```python
from build123d import *

# Parameters (mm, degrees)
F0_W     = 254
F0_H     = 25.0825
F1_DEPTH = 3.175
F2_DEPTH = 22.225
F3_DEPTH = 25.4


# Not quite as in the source:
# - a feature names something its author has since deleted; it is built from what else it names


with BuildPart() as f1:
    # F0 (on Top) → F1 (new body)
    with BuildSketch(Plane.XY):
        with Locations((-10.5066807906, 37.553641122)):
            Rectangle(F0_W, F0_H)
    extrude(amount=F1_DEPTH)



with BuildPart() as f1b:
    # F0 (on Top) → F1, piece 2 (new body)
    with BuildSketch(Plane.XY):
        with Locations((-10.5066807906, 7.391141122)):
            Rectangle(F0_W, F0_H)
    extrude(amount=F1_DEPTH)


with BuildPart() as f1c:
    # F0 (on Top) → F1, piece 3 (new body)
    with BuildSketch(Plane.XY):
        Polygon((-137.5066807906, -61.030108878), (-137.5066807906, -66.110108878), (-112.1066807906, -66.110108878), (-112.1066807906, -61.030108878), (-112.1066807906, -10.230108878), (-137.5066807906, -10.230108878), align=None)
    extrude(amount=F1_DEPTH)


with BuildPart() as f1d:
    # F0 (on Top) → F1, piece 4 (new body)
    with BuildSketch(Plane.XY):
        Polygon((-107.0266807906, -61.030108878), (-107.0266807906, -66.110108878), (-81.6266807906, -66.110108878), (-81.6266807906, -61.030108878), (-81.6266807906, -10.230108878), (-107.0266807906, -10.230108878), align=None)
    extrude(amount=F1_DEPTH)


with BuildPart() as f1e:
    # F0 (on Top) → F1, piece 5 (new body)
    with BuildSketch(Plane.XY):
        Polygon((-76.5466807906, -61.030108878), (-76.5466807906, -66.110108878), (-51.1466807906, -66.110108878), (-51.1466807906, -61.030108878), (-51.1466807906, -10.230108878), (-76.5466807906, -10.230108878), align=None)
    extrude(amount=F1_DEPTH)


with BuildPart() as f1f:
    # F0 (on Top) → F1, piece 6 (new body)
    with BuildSketch(Plane.XY):
        Polygon((-46.0666807906, -61.030108878), (-46.0666807906, -66.110108878), (-20.6666807906, -66.110108878), (-20.6666807906, -61.030108878), (-20.6666807906, -10.230108878), (-46.0666807906, -10.230108878), align=None)
    extrude(amount=F1_DEPTH)


with BuildPart() as f1g:
    # F0 (on Top) → F1, piece 7 (new body)
    with BuildSketch(Plane.XY):
        Polygon((-15.5866807906, -66.110108878), (9.8133192094, -66.110108878), (9.8133192094, -61.030108878), (9.8133192094, -10.230108878), (-15.5866807906, -10.230108878), (-15.5866807906, -61.030108878), align=None)
    extrude(amount=F1_DEPTH)


with BuildPart() as f1h:
    # F0 (on Top) → F1, piece 8 (new body)
    with BuildSketch(Plane.XY):
        Polygon((14.8933192094, -66.110108878), (40.2933192094, -66.110108878), (40.2933192094, -61.030108878), (40.2933192094, -10.230108878), (14.8933192094, -10.230108878), (14.8933192094, -61.030108878), align=None)
    extrude(amount=F1_DEPTH)


with BuildPart() as f1i:
    # F0 (on Top) → F1, piece 9 (new body)
    with BuildSketch(Plane.XY):
        Polygon((45.3733192094, -66.110108878), (70.7733192094, -66.110108878), (70.7733192094, -61.030108878), (70.7733192094, -10.230108878), (45.3733192094, -10.230108878), (45.3733192094, -61.030108878), align=None)
    extrude(amount=F1_DEPTH)


with BuildPart() as f1j:
    # F0 (on Top) → F1, piece 10 (new body)
    with BuildSketch(Plane.XY):
        Polygon((75.8533192094, -66.110108878), (116.4933192094, -66.110108878), (116.4933192094, -61.030108878), (116.4933192094, -10.230108878), (75.8533192094, -10.230108878), (75.8533192094, -61.030108878), align=None)
    extrude(amount=F1_DEPTH)


with BuildPart() as f1_1:
    add(f1.part)

    add(f1b.part)  # F2 merges F1b

    add(f1c.part)  # F2 merges F1c

    add(f1d.part)  # F2 merges F1d

    add(f1e.part)  # F2 merges F1e

    add(f1f.part)  # F2 merges F1f

    add(f1g.part)  # F2 merges F1g

    add(f1h.part)  # F2 merges F1h

    add(f1i.part)  # F2 merges F1i

    add(f1j.part)  # F2 merges F1j
    # F0 (on Top) → F2 (join)
    with BuildSketch(Plane.XY):
        Polygon((121.5733192094, 55.174891122), (-142.5866807906, 55.174891122), (-142.5866807906, -66.110108878), (-137.5066807906, -66.110108878), (-137.5066807906, -61.030108878), (-137.5066807906, -10.230108878), (-112.1066807906, -10.230108878), (-107.0266807906, -10.230108878), (-81.6266807906, -10.230108878), (-76.5466807906, -10.230108878), (-51.1466807906, -10.230108878), (-46.0666807906, -10.230108878), (-20.6666807906, -10.230108878), (-15.5866807906, -10.230108878), (9.8133192094, -10.230108878), (14.8933192094, -10.230108878), (40.2933192094, -10.230108878), (45.3733192094, -10.230108878), (70.7733192094, -10.230108878), (75.8533192094, -10.230108878), (116.4933192094, -10.230108878), (116.4933192094, -61.030108878), (116.4933192094, -66.110108878), (121.5733192094, -66.110108878), align=None)
        with Locations((-10.5066807906, 7.391141122)):
            Rectangle(F0_W, F0_H, mode=Mode.SUBTRACT)
        with Locations((-10.5066807906, 37.553641122)):
            Rectangle(F0_W, F0_H, mode=Mode.SUBTRACT)
        Polygon((-112.1066807906, -61.030108878), (-112.1066807906, -66.110108878), (-107.0266807906, -66.110108878), (-107.0266807906, -61.030108878), (-107.0266807906, -10.230108878), (-112.1066807906, -10.230108878), align=None)
        Polygon((-81.6266807906, -61.030108878), (-81.6266807906, -66.110108878), (-76.5466807906, -66.110108878), (-76.5466807906, -61.030108878), (-76.5466807906, -10.230108878), (-81.6266807906, -10.230108878), align=None)
        Polygon((-51.1466807906, -61.030108878), (-51.1466807906, -66.110108878), (-46.0666807906, -66.110108878), (-46.0666807906, -61.030108878), (-46.0666807906, -10.230108878), (-51.1466807906, -10.230108878), align=None)
        Polygon((-20.6666807906, -61.030108878), (-20.6666807906, -66.110108878), (-15.5866807906, -66.110108878), (-15.5866807906, -61.030108878), (-15.5866807906, -10.230108878), (-20.6666807906, -10.230108878), align=None)
        Polygon((9.8133192094, -66.110108878), (14.8933192094, -66.110108878), (14.8933192094, -61.030108878), (14.8933192094, -10.230108878), (9.8133192094, -10.230108878), (9.8133192094, -61.030108878), align=None)
        Polygon((40.2933192094, -66.110108878), (45.3733192094, -66.110108878), (45.3733192094, -61.030108878), (45.3733192094, -10.230108878), (40.2933192094, -10.230108878), (40.2933192094, -61.030108878), align=None)
        Polygon((70.7733192094, -66.110108878), (75.8533192094, -66.110108878), (75.8533192094, -61.030108878), (75.8533192094, -10.230108878), (70.7733192094, -10.230108878), (70.7733192094, -61.030108878), align=None)
    extrude(amount=F2_DEPTH)

    # F3 (cut): faces of the model
    f3_faces = [f1_1.faces().sort_by_distance(p)[0] for p in [
        (-137.5066807906, 7.391141122, 12.7),
        (-137.5066807906, 37.553641122, 12.7),
    ]]
    extrude(f3_faces, amount=-F3_DEPTH, mode=Mode.SUBTRACT)


solid = f1_1.part
```
Can you work these out from the model? Positions are in its coordinate system, mm. A direction names the side the tool comes from. Round coordinates to 2 decimals unless told otherwise and drop trailing zeros. Order: outer loops, then holes, each group sorted by start corner. A loop starts at its lowest first (then second) coordinate and runs counter-clockwise, first axis right, second up. Notation, with made-up numbers: (76.25, 43) -> (100.25, 43) arc R32 ccw to (100.25, 81) -> close; hole circle Ø8 at (33.5, -15). An arc over 180 degrees is marked (long way). Return JSON: item names as keys, results as strings. Group by question number.
1. If we section it at A-A, the plane x = -68: Write out the boundary of the cut face in (y, z) (3 decimals), then the cut area to 3 significant figures.
2. Will these pins go through, and if not, where does the flat tip stop? pin 1 (12.5 mm diameter, centred on x = -64.5, y = -44.5, fed in from +Z) (3 decimals); pin 2 (5.5 mm diameter, centred on x = -126.5, z = 8.5, fed in from -Y).
3. I need wall thicknesses on line 1 (Y direction, x = -32.5, z = 14); line 2 (Y direction, x = -18.5, z = 9); line 3 (Z direction, x = -57, y = -3.5) (3 decimals). Which ranges of each line are inside material? Lowest first, please. Write a range as [from, to].
4. If we section it at B-B, the plane y = 1.5: Write out the boundary of the cut face in (x, z) (3 decimals).
5. Which directions (+Z, -Z, +X, -X, +Y, -Y) give clear straight access to the entire face, cutting with the end or side of a thin tool? Please do faces 5 (the face through (-9, 55.175, 11)), 6 (the face through (70.773, -38, 13)).
6. We'd pull the mould along Y, two halves only. Please class faces 1 (the face through (-125, -10.23, 13)), 2 (the face through (116.493, 37, 13)), 3 (the face through (-34, -38, 3.175)), 4 (the face through (-11, 7, 3.175)): released by +Y, released by -Y, zero draft, split by the parting line, or undercut.
Output values:
{
 "1": {"outline": "(-66.11, 0) -> (55.175, 0) -> (55.175, 22.225) -> (50.095, 22.225) -> (50.095, 3.175) -> (25.012, 3.175) -> (25.012, 22.225) -> (19.932, 22.225) -> (19.932, 3.175) -> (-5.15, 3.175) -> (-5.15, 22.225) -> (-10.23, 22.225) -> (-10.23, 3.175) -> (-66.11, 3.175) -> close", "area": "675 mm²"},
 "2": {"pin 1": "z = 3.175", "pin 2": "y = -10.23"},
 "3": {"line 1": "[-10.23, -5.15], [19.93, 25.01], [50.09, 55.17]", "line 2": "[-66.11, -5.15], [19.93, 25.01], [50.09, 55.17]", "line 3": "[0, 3.175]"},
 "4": {"outline": "(-142.587, 0) -> (121.573, 0) -> (121.573, 22.225) -> (116.493, 22.225) -> (116.493, 3.175) -> (-142.587, 3.175) -> close"},
 "5": {"face 5": "+Z, -Z, +X, -X, +Y", "face 6": "+Z, -Y"},
 "6": {"face 1": "released by -Y", "face 2": "undercut", "face 3": "zero draft", "face 4": "undercut"}
}
